from build123d import *

# Parameters (mm, degrees)
SKETCH_1_W           = 174.15
SKETCH_1_H           = 108
EXTRUDE_1_DEPTH      = 63
CUT_EXTRUDE_2_DEPTH  = 174.15
CUT_EXTRUDE_3_REACH  = 122.279
SKETCH_6_W           = 2
SKETCH_6_H           = 108
SKETCH_7_W           = 96
SKETCH_7_H           = 50.25
CUT_EXTRUDE_5_DEPTH  = 168.15
SKETCH_8_W           = 87.5
SKETCH_8_H           = 4.75
CUT_EXTRUDE_6_DEPTH  = 168.15
SKETCH_10_W          = 168.15
SKETCH_10_H          = 87.5
CUT_EXTRUDE_8_DEPTH  = 59
SKETCH_12_W          = 168.15
SKETCH_12_H          = 96
EXTRUDE_2_DEPTH      = 2
SKETCH_15_W          = 25
SKETCH_15_H          = 70
SKETCH_15_W_2        = 55
SKETCH_15_H_2        = 20
SKETCH_15_W_3        = 44.398131355
SKETCH_15_H_3        = 87.5
CUT_EXTRUDE_9_DEPTH  = 2
SKETCH_16_W          = 25
SKETCH_16_H          = 96
SKETCH_16_W_2        = 32.283516817
CUT_EXTRUDE_10_DEPTH = 2
SKETCH_17_W          = 2
SKETCH_17_H          = 96
EXTRUDE_3_DEPTH      = 5
SKETCH_18_W          = 2
SKETCH_18_H          = 87.5
EXTRUDE_4_DEPTH      = 5
SKETCH_19_W          = 100
SKETCH_19_H          = 18
CUT_EXTRUDE_11_DEPTH = 6
SKETCH_23_W          = 65.205598619
SKETCH_23_H          = 48.744694075
CUT_EXTRUDE_13_DEPTH = 2
CUT_EXTRUDE_START    = -63
CUT_EXTRUDE_14_DEPTH = 63
SKETCH_28_W          = 2
SKETCH_28_H          = 4.25
EXTRUDE_6_DEPTH      = 4.75
SKETCH_31_W          = 13
SKETCH_31_H          = 55
CUT_EXTRUDE_15_DEPTH = 10
SKETCH_34_W          = 103.070926165
SKETCH_34_H          = 3
CUT_EXTRUDE_16_DEPTH = 143.15
SKETCH_37_W          = 96
SKETCH_37_H          = 4
CUT_EXTRUDE_17_DEPTH = 10
SKETCH_38_W          = 123.751868645
SKETCH_38_H          = 87.5
CUT_EXTRUDE_18_DEPTH = 10
CUT_EXTRUDE_20_REACH = 194.907
SKETCH_42_W          = 103.070926165
SKETCH_42_H          = 3
SKETCH_45_W          = 100.033953054
SKETCH_45_H          = 3
CUT_EXTRUDE_21_DEPTH = 6
SKETCH_46_W          = 15.60461182
SKETCH_46_H          = 6
EXTRUDE_7_DEPTH      = 21
SKETCH_47_W          = 100.033953054
SKETCH_47_H          = 22
CUT_EXTRUDE_22_DEPTH = 2
SKETCH_48_W          = 87.5
SKETCH_48_H          = 5
CUT_EXTRUDE_23_DEPTH = 2
SKETCH_49_W          = 108
SKETCH_49_H          = 6.75
CUT_EXTRUDE_24_DEPTH = 2
EXTRUDE_8_DEPTH      = 2
SKETCH_54_W          = 0.5
SKETCH_54_H          = 0.5
EXTRUDE_10_DEPTH     = 65.205598619
EXTRUDE_11_REACH     = 158.761
SKETCH_55_W          = 0.5
SKETCH_55_H          = 0.5


with BuildPart() as part:
    # 스케치1 → 보스-돌출1 (new body)
    with BuildSketch(Plane(origin=(0, 0, 0), x_dir=(1, 0, 0), z_dir=(0, 1, 0))):
        Rectangle(SKETCH_1_W, SKETCH_1_H)
    extrude(amount=EXTRUDE_1_DEPTH)

    # 스케치5 → 컷-돌출2 (cut)
    with BuildSketch(Plane.ZY.offset(87.075)):
        Polygon((-48, 0), (-47.75, 0), (-47.75, 2.75), (-45.75, 2.75), (-45.75, 4.75), (-52.25, 4.75), (-52.25, 2.75), (-50.25, 2.75), (-50.25, 0), (-50, 0), (-50, 3), (-52, 3), (-52, 4.5), (-46, 4.5), (-46, 3), (-48, 3), align=None)
        Polygon((-50, 0), (-48, 0), (-48, 3), (-46, 3), (-46, 4.5), (-52, 4.5), (-52, 3), (-50, 3), align=None)
        Polygon((50, 3), (50, 0), (50.25, 0), (50.25, 2.75), (52.25, 2.75), (52.25, 4.75), (45.75, 4.75), (45.75, 2.75), (47.75, 2.75), (47.75, 0), (48, 0), (48, 3), (46, 3), (46, 4.5), (52, 4.5), (52, 3), align=None)
        Polygon((48, 0), (50, 0), (50, 3), (52, 3), (52, 4.5), (46, 4.5), (46, 3), (48, 3), align=None)
    extrude(amount=-CUT_EXTRUDE_2_DEPTH, mode=Mode.SUBTRACT)

    # 컷-돌출3: up to this face of the body (flat: up to its plane)
    cut_extrude_3_end = Plane(part.part.faces().sort_by_distance((0, 4.75, 49))[0])
    # 스케치6 → 컷-돌출3 (cut, up to the picked face)
    with BuildSketch(Plane.XZ, mode=Mode.PRIVATE) as cut_extrude_3_sk1:
        with Locations((-86.075, 0)):
            Rectangle(SKETCH_6_W, SKETCH_6_H)
    cut_extrude_3_tool1 = split(extrude(cut_extrude_3_sk1.sketch, amount=-CUT_EXTRUDE_3_REACH, mode=Mode.PRIVATE), bisect_by=cut_extrude_3_end, keep=Keep.BOTH, mode=Mode.PRIVATE)
    add(cut_extrude_3_tool1.solids().sort_by(Axis((-86.075, 0, 0), (0, 1, 0)))[0], mode=Mode.SUBTRACT)

    # 스케치7 → 컷-돌출5 (cut)
    with BuildSketch(Plane(origin=(87.075, 0, 0), x_dir=(0, 0, -1), z_dir=(1, 0, 0))):
        with Locations((0, 31.875)):
            Rectangle(SKETCH_7_W, SKETCH_7_H)
    extrude(amount=-CUT_EXTRUDE_5_DEPTH, mode=Mode.SUBTRACT)

    # 스케치8 → 컷-돌출6 (cut)
    with BuildSketch(Plane(origin=(87.075, 0, 0), x_dir=(0, 0, -1), z_dir=(1, 0, 0))):
        with Locations((0, 4.375)):
            Rectangle(SKETCH_8_W, SKETCH_8_H)
    extrude(amount=-CUT_EXTRUDE_6_DEPTH, mode=Mode.SUBTRACT)

    # 스케치10 → 컷-돌출8 (cut)
    with BuildSketch(Plane(origin=(0, 2, 0), x_dir=(1, 0, 0), z_dir=(0, 1, 0))):
        with Locations((3, 0)):
            Rectangle(SKETCH_10_W, SKETCH_10_H)
    extrude(amount=CUT_EXTRUDE_8_DEPTH, mode=Mode.SUBTRACT)

    # 스케치12 → 보스-돌출2 (add)
    with BuildSketch(Plane(origin=(0, 24, 0), x_dir=(-1, 0, 0), z_dir=(0, -1, 0))):
        with Locations((-3, 0)):
            Rectangle(SKETCH_12_W, SKETCH_12_H)
    extrude(amount=EXTRUDE_2_DEPTH)

    # 스케치15 → 컷-돌출9 (cut)
    with BuildSketch(Plane(origin=(0, 2, 0), x_dir=(1, 0, 0), z_dir=(0, 1, 0))):
        with Locations((-68.575, 8.75)):
            Rectangle(SKETCH_15_W, SKETCH_15_H)
        with Locations((-9.233175572, -33.75)):
            Rectangle(SKETCH_15_W_2, SKETCH_15_H_2)
        with Locations((64.875934323, 0)):
            Rectangle(SKETCH_15_W_3, SKETCH_15_H_3)
    extrude(amount=-CUT_EXTRUDE_9_DEPTH, mode=Mode.SUBTRACT)

    # 스케치16 → 컷-돌출10 (cut)
    with BuildSketch(Plane(origin=(0, 24, 0), x_dir=(1, 0, 0), z_dir=(0, 1, 0))):
        with Locations((-68.575, 0)):
            Rectangle(SKETCH_16_W, SKETCH_16_H)
        with Locations((70.933241592, 0)):
            Rectangle(SKETCH_16_W_2, SKETCH_16_H)
    extrude(amount=-CUT_EXTRUDE_10_DEPTH, mode=Mode.SUBTRACT)

    # 스케치17 → 보스-돌출3 (add)
    with BuildSketch(Plane(origin=(0, 24, 0), x_dir=(1, 0, 0), z_dir=(0, 1, 0))):
        with Locations((-55.075, 0)):
            Rectangle(SKETCH_17_W, SKETCH_17_H)
    extrude(amount=EXTRUDE_3_DEPTH)

    # 스케치18 → 보스-돌출4 (add)
    with BuildSketch(Plane(origin=(0, 2, 0), x_dir=(1, 0, 0), z_dir=(0, 1, 0))):
        with Locations((-55.075, 0)):
            Rectangle(SKETCH_18_W, SKETCH_18_H)
    extrude(amount=EXTRUDE_4_DEPTH)

    # 스케치19 → 컷-돌출11 (cut)
    with BuildSketch(Plane(origin=(0, 0, 48), x_dir=(-1, 0, 0), z_dir=(0, 0, -1))):
        with Locations((4.075, 38)):
            Rectangle(SKETCH_19_W, SKETCH_19_H)
    extrude(amount=-CUT_EXTRUDE_11_DEPTH, mode=Mode.SUBTRACT)

    # 스케치23 → 컷-돌출13 (cut)
    with BuildSketch(Plane(origin=(0, 63, 0), x_dir=(1, 0, 0), z_dir=(0, 1, 0))):
        with Locations((-5.140341164, 12.481591832)):
            Rectangle(SKETCH_23_W, SKETCH_23_H)
    extrude(amount=-CUT_EXTRUDE_13_DEPTH, mode=Mode.SUBTRACT)

    # 스케치26 → 컷-돌출14 (cut)
    with BuildSketch(Plane(origin=(0, 63, 0), x_dir=(1, 0, 0), z_dir=(0, 1, 0)).offset(CUT_EXTRUDE_START)):
        Polygon((82.075, 52), (85.075, 52), (85.075, 48), (87.075, 48), (87.075, -48), (85.075, -48), (85.075, -52), (82.075, -52), align=None)
    extrude(amount=CUT_EXTRUDE_14_DEPTH, mode=Mode.SUBTRACT)

    # 스케치28 → 보스-돌출6 (add)
    with BuildSketch(Plane.XZ.offset(-4.75)):
        with Locations((86.075, 50.125)):
            Rectangle(SKETCH_28_W, SKETCH_28_H)
        with Locations((86.075, -50.125)):
            Rectangle(SKETCH_28_W, SKETCH_28_H)
    extrude(amount=EXTRUDE_6_DEPTH)

    # 스케치31 → 컷-돌출15 (cut)
    with BuildSketch(Plane(origin=(0, 63, 0), x_dir=(1, 0, 0), z_dir=(0, 1, 0))):
        with Locations((75.575, 0)):
            Rectangle(SKETCH_31_W, SKETCH_31_H)
    extrude(amount=-CUT_EXTRUDE_15_DEPTH, mode=Mode.SUBTRACT)

    # 스케치34 → 컷-돌출16 (cut)
    with BuildSketch(Plane(origin=(87.075, 0, 0), x_dir=(0, 0, -1), z_dir=(1, 0, 0))):
        with Locations((-0.464536917, 23.5)):
            Rectangle(SKETCH_34_W, SKETCH_34_H)
    extrude(amount=-CUT_EXTRUDE_16_DEPTH, mode=Mode.SUBTRACT)

    # 스케치37 → 컷-돌출17 (cut)
    with BuildSketch(Plane(origin=(-54.075, 0, 0), x_dir=(0, 0, -1), z_dir=(1, 0, 0))):
        with Locations((0, 27)):
            Rectangle(SKETCH_37_W, SKETCH_37_H)
    extrude(amount=-CUT_EXTRUDE_17_DEPTH, mode=Mode.SUBTRACT)

    # 스케치38 → 컷-돌출18 (cut)
    with BuildSketch(Plane(origin=(0, 2, 0), x_dir=(1, 0, 0), z_dir=(0, 1, 0))):
        with Locations((-19.199065677, 0)):
            Rectangle(SKETCH_38_W, SKETCH_38_H)
    extrude(amount=-CUT_EXTRUDE_18_DEPTH, mode=Mode.SUBTRACT)

    # 컷-돌출20: up to this face of the body (flat: up to its plane)
    cut_extrude_20_end = Plane(part.part.faces().sort_by_distance((-56.075, 23.5, -49.535463082))[0])
    # 스케치42 → 컷-돌출20 (cut, up to the picked face)
    with BuildSketch(Plane(origin=(87.075, 0, 0), x_dir=(0, 0, -1), z_dir=(1, 0, 0)), mode=Mode.PRIVATE) as cut_extrude_20_sk1:
        with Locations((-0.464536917, 17.5)):
            Rectangle(SKETCH_42_W, SKETCH_42_H)
    cut_extrude_20_tool1 = split(extrude(cut_extrude_20_sk1.sketch, amount=-CUT_EXTRUDE_20_REACH, mode=Mode.PRIVATE), bisect_by=cut_extrude_20_end, keep=Keep.BOTH, mode=Mode.PRIVATE)
    add(cut_extrude_20_tool1.solids().sort_by(Axis((87.075, 17.5, 0.464537), (-1, 0, 0)))[0], mode=Mode.SUBTRACT)

    # 스케치45 → 컷-돌출21 (cut)
    with BuildSketch(Plane(origin=(0, 0, 48), x_dir=(-1, 0, 0), z_dir=(0, 0, -1))):
        with Locations((4.091976527, 27.5)):
            Rectangle(SKETCH_45_W, SKETCH_45_H)
    extrude(amount=-CUT_EXTRUDE_21_DEPTH, mode=Mode.SUBTRACT)

    # 스케치46 → 보스-돌출7 (add)
    with BuildSketch(Plane(origin=(0, 26, 0), x_dir=(1, 0, 0), z_dir=(0, 1, 0))):
        with Locations((24.337049492, -51)):
            Rectangle(SKETCH_46_W, SKETCH_46_H)
    extrude(amount=EXTRUDE_7_DEPTH)

    # 스케치47 → 컷-돌출22 (cut)
    with BuildSketch(Plane(origin=(0, 0, 48), x_dir=(-1, 0, 0), z_dir=(0, 0, -1))):
        with Locations((4.091976527, 36)):
            Rectangle(SKETCH_47_W, SKETCH_47_H)
    extrude(amount=-CUT_EXTRUDE_22_DEPTH, mode=Mode.SUBTRACT)

    # 스케치48 → 컷-돌출23 (cut)
    with BuildSketch(Plane(origin=(-54.075, 0, 0), x_dir=(0, 0, -1), z_dir=(1, 0, 0))):
        with Locations((0, 4.5)):
            Rectangle(SKETCH_48_W, SKETCH_48_H)
    extrude(amount=-CUT_EXTRUDE_23_DEPTH, mode=Mode.SUBTRACT)

    # 스케치49 → 컷-돌출24 (cut)
    with BuildSketch(Plane(origin=(87.075, 0, 0), x_dir=(0, 0, -1), z_dir=(1, 0, 0))):
        with Locations((0, 3.375)):
            Rectangle(SKETCH_49_W, SKETCH_49_H)
    extrude(amount=-CUT_EXTRUDE_24_DEPTH, mode=Mode.SUBTRACT)

    # 스케치51 → 보스-돌출8 (add)
    with BuildSketch(Plane.ZY.offset(85.075)):
        Polygon((52.25, 2.75), (50.25, 2.75), (50.25, 0), (54, 0), (54, 4.75), (52.25, 4.75), align=None)
        Polygon((-52.25, 2.75), (-52.25, 4.75), (-54, 4.75), (-54, 0), (-50.25, 0), (-50.25, 2.75), align=None)
        Polygon((47.75, 2.75), (45.75, 2.75), (45.75, 4.75), (-45.75, 4.75), (-45.75, 2.75), (-47.75, 2.75), (-47.75, 0), (47.75, 0), align=None)
    extrude(amount=EXTRUDE_8_DEPTH)

    # 스케치54 → 보스-돌출10 (add)
    with BuildSketch(Plane(origin=(-37.743140474, 0, 0), x_dir=(0, 0, -1), z_dir=(1, 0, 0))):
        with Locations((-10.286427881, 62)):
            Rectangle(SKETCH_54_W, SKETCH_54_H)
        with Locations((-0.286427881, 62)):
            Rectangle(SKETCH_54_W, SKETCH_54_H)
        with Locations((9.713572119, 62)):
            Rectangle(SKETCH_54_W, SKETCH_54_H)
        with Locations((19.713572119, 62)):
            Rectangle(SKETCH_54_W, SKETCH_54_H)
        with Locations((29.713572119, 62)):
            Rectangle(SKETCH_54_W, SKETCH_54_H)
    extrude(amount=EXTRUDE_10_DEPTH)

    # 보스-돌출11: up to this face of the body (flat: up to its plane)
    extrude_11_end = Plane(part.part.faces().sort_by_distance((-87.075, 31.667900174, 0))[0])
    # 스케치55 → 보스-돌출11 (add, up to the picked face)
    with BuildSketch(Plane.ZY.offset(-45.925), mode=Mode.PRIVATE) as extrude_11_sk1:
        with Locations((51, 44.102500149)):
            Rectangle(SKETCH_55_W, SKETCH_55_H)
    extrude_11_tool1 = split(extrude(extrude_11_sk1.sketch, amount=EXTRUDE_11_REACH, mode=Mode.PRIVATE), bisect_by=extrude_11_end, keep=Keep.BOTH, mode=Mode.PRIVATE)
    # 스케치55 → 보스-돌출11 (add, up to the picked face)
    with BuildSketch(Plane.ZY.offset(-45.925), mode=Mode.PRIVATE) as extrude_11_sk2:
        with Locations((51, 37.102500149)):
            Rectangle(SKETCH_55_W, SKETCH_55_H)
    extrude_11_tool2 = split(extrude(extrude_11_sk2.sketch, amount=EXTRUDE_11_REACH, mode=Mode.PRIVATE), bisect_by=extrude_11_end, keep=Keep.BOTH, mode=Mode.PRIVATE)
    # 스케치55 → 보스-돌출11 (add, up to the picked face)
    with BuildSketch(Plane.ZY.offset(-45.925), mode=Mode.PRIVATE) as extrude_11_sk3:
        with Locations((51, 30.102500149)):
            Rectangle(SKETCH_55_W, SKETCH_55_H)
    extrude_11_tool3 = split(extrude(extrude_11_sk3.sketch, amount=EXTRUDE_11_REACH, mode=Mode.PRIVATE), bisect_by=extrude_11_end, keep=Keep.BOTH, mode=Mode.PRIVATE)
    add(extrude_11_tool1.solids().sort_by(Axis((45.925, 44.1025, 51), (-1, 0, 0)))[0])
    add(extrude_11_tool2.solids().sort_by(Axis((45.925, 37.1025, 51), (-1, 0, 0)))[0])
    add(extrude_11_tool3.solids().sort_by(Axis((45.925, 30.1025, 51), (-1, 0, 0)))[0])


solid = part.part
For this review, take the finished solid that the model builds, in its own axes (mm). A direction names the side the tool comes from. Coordinates: 2 decimals unless noted, no trailing zeros. Loops run counter-clockwise (first coordinate to the right, second up) from the corner with the lowest first, then second, coordinate; pieces in that order, holes last. Notation, with made-up numbers: (45.5, -22.75) - (94.5, -22.75) arc R17 cw to (94.5, 3.25) - close; hole circle Ø5 at (46.25, 49). An arc over 180 degrees is marked (long way). Use a Markdown table: item, result. Add a question column.
Item 1: We need section D-D (y = 54.5). Give the boundary of the cut face in (x, z) (3 decimals).
Item 2: For line 1 (Z direction, x = 59, y = 58); line 2 (Z direction, x = -4.5, y = 24); line 3 (X direction, y = 52.5, z = 0.5) (3 decimals), list the stretches that pass through material, from the lowest coordinate up.
Item 3: We need section B-B (y = 41). Give the boundary of the cut face in (x, z) (3 decimals), and give its area (3 significant figures).
Item 4: We need section A-A (z = 6). Give the boundary of the cut face in (x, y) (3 decimals), and give its area (3 significant figures).
Item 5: Tool access review of faces 4 (the face through (85.075, 11, 50)), 5 (the face through (39, 26, 52)), 6 (the face through (18, 34, 50)), 7 (the face through (2, 6.75, -46)), 8 (the face through (-1, 59, -43.75)): name each direction out of +Z, -Z, +X, -X, +Y, -Y from which nothing blocks a thin tool from reaching the whole face with its end or side.
Item 6: We need section C-C (z = -34). Give the boundary of the cut face in (x, y) (3 decimals).
Item 7: Insertion check: pin 1 Ø0.6 at (x, y) = (40.5, 37) entering from +Z; pin 2 Ø1 at (x, z) = (62.5, -2.5) entering from -Y; pin 3 Ø1.5 at (y, z) = (17.5, -49.5) entering from +X (3 decimals). Each pin has a flat end and moves straight along its axis. Give the tip position at first contact, or say it passes through.
Item 8: Mouldability with a two-part tool opening along Z and no side actions: class faces 1 (the face through (1, 24, 54)), 2 (the face through (0, 0, -52)), 3 (the face through (-81.075, 31, 1)) as pulls with the +Z half, pulls with the -Z half, needs draft (parallel to the pull), parting line crosses it, or undercut.
Results list:
| question | item | result |
|---|---|---|
| 1 | outline | (-87.075, -54) - (87.075, -54) - (87.075, -48) - (85.075, -48) - (85.075, -52) - (82.075, -52) - (82.075, -48) - (-81.075, -48) - (-81.075, 48) - (82.075, 48) - (82.075, 52) - (85.075, 52) - (85.075, 48) - (87.075, 48) - (87.075, 54) - (-87.075, 54) - close |
| 2 | line 1 | z = -54 to -43.75, 43.75 to 54 |
| 2 | line 2 | z = -54 to -51.07, 52 to 54 |
| 2 | line 3 | x = -87.075 to -81.075 |
| 3 | outline | (-87.075, -54) - (87.075, -54) - (87.075, -48) - (85.075, -48) - (85.075, -52) - (82.075, -52) - (82.075, -48) - (-81.075, -48) - (-81.075, 48) - (-54.109, 48) - (-54.109, 50) - (-54.075, 50) - (-54.075, 54) - (-87.075, 54) - close; (16.535, 50) - (32.139, 50) - (32.139, 54) - (16.535, 54) - close; (45.925, 48) - (82.075, 48) - (82.075, 52) - (85.075, 52) - (85.075, 48) - (87.075, 48) - (87.075, 54) - (45.925, 54) - close |
| 3 | area | 2,100 mm^2 |
| 4 | outline | (-87.075, 0) - (-81.075, 0) - (-81.075, 61) - (-37.743, 61) - (-37.743, 63) - (-87.075, 63) - close; (27.462, 61) - (69.075, 61) - (69.075, 63) - (27.462, 63) - close |
| 4 | area | 548 mm^2 |
| 5 | face 4 | +Y, -Y |
| 5 | face 5 | +Z |
| 5 | face 6 | none |
| 5 | face 7 | +X |
| 5 | face 8 | +X, -Y |
| 6 | outline | (-87.075, 0) - (-81.075, 0) - (-81.075, 61) - (-37.743, 61) - (-37.743, 63) - (-87.075, 63) - close; (27.462, 61) - (82.075, 61) - (82.075, 63) - (27.462, 63) - close |
| 7 | pin 1 | stops at z = 51.25 |
| 7 | pin 2 | stops at y = 61 |
| 7 | pin 3 | stops at x = -56.075 |
| 8 | face 1 | pulls with the +Z half |
| 8 | face 2 | needs draft |
| 8 | face 3 | undercut |
